from build123d import *

# Parameters (mm, degrees)
SKETCH1_W           = 45
SKETCH1_H           = 95.8
BOSS_EXTRUDE1_DEPTH = 13
CUT_EXTRUDE1_DEPTH  = 96.8
FILLET2_R           = 3.5


with BuildPart() as part:
    # Sketch1 → Boss-Extrude1 (new body)
    with BuildSketch(Plane(origin=(0, 0, 0), x_dir=(1, 0, 0), z_dir=(0, 1, 0))):
        Rectangle(SKETCH1_W, SKETCH1_H)
    extrude(amount=BOSS_EXTRUDE1_DEPTH)

    # Sketch15 → Cut-Extrude1 (cut, through all)
    with BuildSketch(Plane.XY.offset(47.9)):
        with BuildLine():
            Line((-15.5, 7), (15.5, 7))
            ThreePointArc((15.5, 7), (20.449747468, 4.949747468), (22.5, 0))
            Line((22.5, 0), (-22.5, 0))
            ThreePointArc((-22.5, 0), (-20.449747468, 4.949747468), (-15.5, 7))
        make_face()
    extrude(amount=-CUT_EXTRUDE1_DEPTH, mode=Mode.SUBTRACT)

    # Fillet2
    fillet2_edges = [part.edges().sort_by_distance(p)[0] for p in [
        (22.5, 13, 0),
        (-22.5, 13, 0),
    ]]
    fillet(fillet2_edges, radius=FILLET2_R)


solid = part.part
Model file for the job. Use its own axes, mm. A direction names the side the tool comes from. Round coordinates to 2 decimals unless told otherwise and drop trailing zeros. Loops run counter-clockwise (first coordinate to the right, second up) from the corner with the lowest first, then second, coordinate; pieces in that order, holes last. Notation, with made-up numbers: (46.5, 34.25) - (54.5, 34.25) arc R11 ccw to (54.5, 53.25) - close; hole circle Ø4 at (-19, 52). An arc over 180 degrees is marked (long way). Write each question's results on one line, items separated by ' | '.
(1) Wall check: L1, parallel to Y at x = 8.5, z = 33; L2, parallel to X at y = 2.5, z = 22; L3, parallel to X at y = 5, z = -33.5. Give the ranges that are in metal, low to high.
Answer below:
L1: y = 7 to 13 | L2: x = -22.5 to -22.04, 22.04 to 22.5 | L3: x = -22.5 to -20.4, 20.4 to 22.5
(2) Saw through at D-D, the plane y = 5.75. List the corners of the cut face in (x, z).
Answer below:
outline: (-22.5, -47.9) - (-19.49, -47.9) - (-19.49, 47.9) - (-22.5, 47.9) - close; (19.49, -47.9) - (22.5, -47.9) - (22.5, 47.9) - (19.49, 47.9) - close
(3) Saw through at C-C, the plane x = 1. List the corners of the cut face in (y, z), then the cut area to 3 significant figures.
Answer below:
outline: (7, -47.9) - (13, -47.9) - (13, 47.9) - (7, 47.9) - close | area: 575 mm^2
(4) 3-axis set-ups, long thin cutter, end or side, ignore diameter. For faces 1 (the cylindrical face through (20.4, 5, 0.7)), 2 (the cylindrical face through (21.45, 12, -0.67)): which of +Z, -Z, +X, -X, +Y, -Y reach the whole face in a straight line?
Answer below:
face 1: +Z, -Z, -Y | face 2: +Z, -Z, +X, +Y
(5) Pin check, flat tips, straight feed: pin 1 (1 mm diameter, centred on x = -5, z = -17.5, fed in from -Y); pin 2 (10 mm diameter, centred on x = -16.5, z = -25, fed in from -Y); pin 3 (6 mm diameter, centred on x = 16.5, z = 28, fed in from -Y). Stop position of each tip, or through.
Answer below:
pin 1: stops at y = 7 | pin 2: stops at y = 3.61 | pin 3: stops at y = 5.74
(6) Saw through at B-B, the plane z = -30. List the corners of the cut face in (x, y), then the cut area to 3 significant figures.
Answer below:
outline: (-22.5, 0) arc R7 cw to (-15.5, 7) - (15.5, 7) arc R7 cw to (22.5, 0) - (22.5, 9.5) arc R3.5 ccw to (19, 13) - (-19, 13) arc R3.5 ccw to (-22.5, 9.5) - close | area: 286 mm^2
(7) Saw through at A-A, the plane y = 2. List the corners of the cut face in (x, z).
Answer below:
outline: (-22.5, -47.9) - (-22.21, -47.9) - (-22.21, 47.9) - (-22.5, 47.9) - close; (22.21, -47.9) - (22.5, -47.9) - (22.5, 47.9) - (22.21, 47.9) - close
